Verification items for the finished model (mm, model axes). A direction names the side the tool comes from. Coordinates: 2 decimals unless noted, no trailing zeros. Order: outer loops, then holes, each group sorted by start corner. A loop starts at its lowest first (then second) coordinate and runs counter-clockwise, first axis right, second up. Notation, with made-up numbers: M -23,84.25 L -1,84.25 A15 cw -1,109.25 Z; hole C 75.5,-21 d10. An arc over 180 degrees is marked long. Write item = value, one per line.
```python
from build123d import *

# Parameters (mm, degrees)
SKETCH_W      = 102.2
SKETCH_H      = 83
SKETCH_W_2    = 30
SKETCH_H_2    = 5
SKETCH_W_3    = 2
SKETCH_H_3    = 25
PAD_DEPTH     = 2
SKETCH001_R   = 2.4
SKETCH001_R_2 = 1.2
PAD001_DEPTH  = 6.2
PAD002_DEPTH  = 6.9
PAD003_DEPTH  = 1
SKETCH004_W   = 1.45
SKETCH004_H   = 11.2
PAD004_DEPTH  = 5
SKETCH005_W   = 1.45
SKETCH005_H   = 5
PAD005_DEPTH  = 11.9
PAD006_DEPTH  = 5


with BuildPart() as part:
    # Sketch → Pad (new body)
    with BuildSketch(Plane.XY):
        Rectangle(SKETCH_W, SKETCH_H)
        with Locations((34.1, 17.5)):
            Rectangle(SKETCH_W_2, SKETCH_H_2, mode=Mode.SUBTRACT)
        with Locations((-34.1, 17.5)):
            Rectangle(SKETCH_W_2, SKETCH_H_2, mode=Mode.SUBTRACT)
        with Locations((6, -27)):
            Rectangle(SKETCH_W_3, SKETCH_H_3, mode=Mode.SUBTRACT)
        with Locations((-6, -27)):
            Rectangle(SKETCH_W_3, SKETCH_H_3, mode=Mode.SUBTRACT)
    extrude(amount=PAD_DEPTH)

    # Sketch001 (on Face22 of Pad) → Pad001 (join)
    with BuildSketch(Plane.XY.offset(2)):
        with Locations((-42.5, -25)):
            Circle(SKETCH001_R)
        with Locations((-42.5, -25)):
            Circle(SKETCH001_R_2, mode=Mode.SUBTRACT)
        with Locations((42.5, 25)):
            Circle(SKETCH001_R)
        with Locations((42.5, 25)):
            Circle(SKETCH001_R_2, mode=Mode.SUBTRACT)
    extrude(amount=PAD001_DEPTH)

    # Sketch002 → Pad002 (join)
    with BuildSketch(Plane.XY):
        Polygon((-51.1, 41.5), (51.1, 41.5), (51.1, 5.05), (53.5, 5.05), (53.5, 43.85), (-53.5, 43.85), (-53.5, 5.05), (-51.1, 5.05), align=None)
    pad002 = extrude(amount=PAD002_DEPTH)

    # Mirrored: Pad002 across XZ
    add(pad002.mirror(Plane.XZ))

    # Sketch003 (on Face36 of Mirrored) → Pad003 (join)
    with BuildSketch(Plane.XY.offset(6.9)):
        Polygon((-51.1, 5.05), (-51.1, 41.5), (51.1, 41.5), (51.1, 5.05), (52.1, 5.05), (52.1, 42.5), (-52.1, 42.5), (-52.1, 5.05), align=None)
    pad003 = extrude(amount=PAD003_DEPTH)

    # Mirrored001: Pad003 across XZ
    add(pad003.mirror(Plane.XZ))

    # Sketch004 (on Face3 of Mirrored001) → Pad004 (join)
    with BuildSketch(Plane.XY.offset(2)):
        with Locations((50.375, 0)):
            Rectangle(SKETCH004_W, SKETCH004_H)
    pad004 = extrude(amount=PAD004_DEPTH)

    # Mirrored002: Pad004 across YZ
    add(pad004.mirror(Plane.YZ))

    # Sketch005 (on Face40 of Mirrored002) → Pad005 (join)
    with BuildSketch(Plane.XY.offset(7)):
        with Locations((50.375, 0)):
            Rectangle(SKETCH005_W, SKETCH005_H)
    pad005 = extrude(amount=PAD005_DEPTH)

    # Mirrored003: Pad005 across YZ
    add(pad005.mirror(Plane.YZ))

    # Sketch006 (on Face2 of Mirrored003) → Pad006 (join)
    with BuildSketch(Plane.XZ.offset(2.5)):
        Polygon((49.65, 18.9), (51.1, 18.9), (53.1, 18.9), (53.1, 19.9), (51.15, 22.9), (49.65, 22.9), align=None)
    pad006 = extrude(amount=-PAD006_DEPTH)

    # Mirrored004: Pad006 across YZ
    add(pad006.mirror(Plane.YZ))


solid = part.part
```
Item 1: Sectioned sample at B-B, the plane z = 16.25. Enter the section's corners in (x, y).
Report:
outline = M -51.1,-2.5 L -49.65,-2.5 L -49.65,2.5 L -51.1,2.5 Z; M 49.65,-2.5 L 51.1,-2.5 L 51.1,2.5 L 49.65,2.5 Z
Item 2: Sectioned sample at A-A, the plane y = -31. Enter the section's corners in (x, z).
Report:
outline = M -53.5,0 L -7,0 L -7,2 L -51.1,2 L -51.1,7.9 L -52.1,7.9 L -52.1,6.9 L -53.5,6.9 Z; M -5,0 L 5,0 L 5,2 L -5,2 Z; M 7,0 L 53.5,0 L 53.5,6.9 L 52.1,6.9 L 52.1,7.9 L 51.1,7.9 L 51.1,2 L 7,2 Z
Item 3: Gauge pin test, flat ends, axial feed: pin 1 (1.1 mm diameter, centred on x = -20.5, z = 7.5, fed in from +Y); pin 2 (1.1 mm diameter, centred on y = 0.5, z = 19.5, fed in from -X); pin 3 (0.5 mm diameter, centred on y = -25.5, z = 7.5, fed in from -X); pin 4 (5 mm diameter, centred on y = -32.5, z = 8.5, fed in from -X). Record the tip position at first contact, or that the pin passes through.
Report:
pin_1 = 42.5
pin_2 = -53.1
pin_3 = -52.1
pin_4 = -53.5
Item 4: Scan lines: L1, parallel to Y at x = -42.5, z = 6.25; L2, parallel to X at y = -35, z = 1.25; L3, parallel to Y at x = 42.5, z = 3.5. Record each from-to range of solid material in increasing order. Write a range as from..to.
Report:
L1 = -43.85..-41.5, -27.4..-26.2, -23.8..-22.6, 41.5..43.85
L2 = -53.5..-7, -5..5, 7..53.5
L3 = -43.85..-41.5, 22.6..23.8, 26.2..27.4, 41.5..43.85
Item 5: Release check for a two-part mould opening along Y. For faces 5 (the cylindrical face through (-41.39, -25.46, 5.06)), 6 (the flat face through (-44, -25, 8.2)) record: pulls with the +Y half, pulls with the -Y half, needs draft (parallel to the pull), parting line crosses it, or undercut.
Report:
face_5 = undercut
face_6 = needs draft
Item 6: Sectioned sample at C-C, the plane x = -42.5. Enter the section's corners in (y, z).
Report:
outline = M -43.85,0 L 15,0 L 15,2 L -22.6,2 L -22.6,8.2 L -23.8,8.2 L -23.8,2 L -26.2,2 L -26.2,8.2 L -27.4,8.2 L -27.4,2 L -41.5,2 L -41.5,7.9 L -42.5,7.9 L -42.5,6.9 L -43.85,6.9 Z; M 20,0 L 43.85,0 L 43.85,6.9 L 42.5,6.9 L 42.5,7.9 L 41.5,7.9 L 41.5,2 L 20,2 Z
Item 7: Tool access check on faces 1 (the flat face through (-1, 41.5, 5)), 2 (the flat face through (51.1, 0, 7)), 3 (the flat face through (52, -5.05, 4)), 4 (the flat face through (-52, 5.05, 4)). Record the directions out of +Z, -Z, +X, -X, +Y, -Y that give a thin tool (end or side, any length) a straight path to the whole face; none if there is none.
Report:
face_1 = +Z
face_2 = -Z, +X
face_3 = +Z, -Z, +X
face_4 = +Z, -Z, -X
Item 8: Sectioned sample at D-D, the plane y = -10.5. Enter the section's corners in (x, z), then the cut area to 3 significant figures.
Report:
outline = M -53.5,0 L 53.5,0 L 53.5,6.9 L 52.1,6.9 L 52.1,7.9 L 51.1,7.9 L 51.1,2 L -51.1,2 L -51.1,7.9 L -52.1,7.9 L -52.1,6.9 L -53.5,6.9 Z
area = 240 mm^2
